```python
from build123d import *

# Parameters (mm, degrees)
F0_W     = 12
F0_H     = 12
F1_DEPTH = 5
F3_DEPTH = 2.5
F5_D     = 7


with BuildPart() as f1:
    # F0 (on Top) → F1 (new body)
    with BuildSketch(Plane.XY):
        Rectangle(F0_W, F0_H)
    extrude(amount=F1_DEPTH)

    # F2 (on face) → F3 (cut)
    with BuildSketch(Plane.XY.offset(5)):
        Polygon((2.453739, -4.25), (4.907477, 0), (2.453739, 4.25), (-2.453739, 4.25), (-4.907477, 0), (-2.453739, -4.25), align=None)
    extrude(amount=-F3_DEPTH, mode=Mode.SUBTRACT)

    # F5 (through all)
    with Locations(Plane.XY.offset(2.5)):
        with Locations((0, 0)):
            Hole(F5_D / 2)


solid = f1.part
```
Could you check a few things on this model? Use its own coordinates, in mm. A direction names the side the tool comes from. Give positions to 0.01 mm unless a question says otherwise; leave off trailing zeros. Order: outer loops, then holes, each group sorted by start corner. A loop starts at its lowest first (then second) coordinate and runs counter-clockwise, first axis right, second up.
Q1. We'd pull the mould along X, two halves only. Please class faces 3 (the flat face through (0, -4.25, 4)), 4 (the flat face through (3.698, 2.095, 3.768)), 5 (the flat face through (-6, 0, 2)), 6 (the flat face through (-3, 4, 5)): +X half, -X half, draft (parallel to the pull), parting line (faces both ways), or undercut.
Q2. Suppose I cut it at A-A, the plane x = 0. Write out the boundary of the cut face in (y, z).
Q3. If I drill on line 1 along Y through (x, z) = (0, 1.65); line 2 along Y through (x, z) = (0.25, 4.75); line 3 along Z through (x, y) = (3.75, 1.25), over which ranges is the centre line in solid material (lowest first)?
Q4. Suppose I cut it at C-C, the plane y = -2.25. Write out the boundary of the cut face in (x, z), and give its area (3 significant figures).
Q5. Suppose I cut it at B-B, the plane z = 4. Write out the boundary of the cut face in (x, y).
Q6. For faces 1 (the flat face through (0, -6, 2)), 2 (the flat face through (0, 4.25, 4)), which set-ups out of +Z, -Z, +X, -X, +Y, -Y let a thin tool reach every point of the face, with its end or its side?
Q7. Suppose I cut it at D-D, the plane z = 1.85. Write out the boundary of the cut face in (x, y).
Solution:
1. face 3: undercut
1. face 4: undercut
1. face 5: -X half
1. face 6: draft
2. outline: (-6, 0) - (-3.5, 0) - (-3.5, 2.5) - (-4.25, 2.5) - (-4.25, 5) - (-6, 5) - close; (3.5, 0) - (6, 0) - (6, 5) - (4.25, 5) - (4.25, 2.5) - (3.5, 2.5) - close
3. line 1: y = -6 to -3.5, 3.5 to 6
3. line 2: y = -6 to -4.25, 4.25 to 6
3. line 3: z = 0 to 2.5
4. outline: (-6, 0) - (-2.68, 0) - (-2.68, 2.5) - (-3.61, 2.5) - (-3.61, 5) - (-6, 5) - close; (2.68, 0) - (6, 0) - (6, 5) - (3.61, 5) - (3.61, 2.5) - (2.68, 2.5) - close
4. area: 28.6 mm2
5. outline: (-6, -6) - (6, -6) - (6, 6) - (-6, 6) - close; hole (-4.91, 0) - (-2.45, -4.25) - (2.45, -4.25) - (4.91, 0) - (2.45, 4.25) - (-2.45, 4.25) - close
6. face 1: +Z, -Z, +X, -X, -Y
6. face 2: +Z
7. outline: (-6, -6) - (6, -6) - (6, 6) - (-6, 6) - close; hole circle Ø7 at (0, 0)
